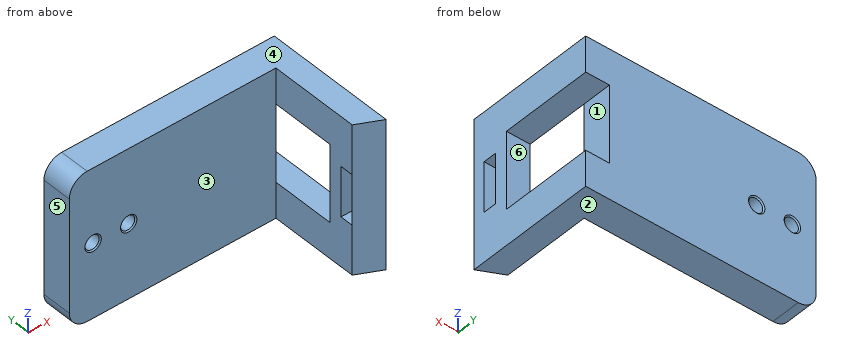
```python
from build123d import *

# Parameters (mm, degrees)
SKETCH1_W             = 44.196
SKETCH1_H             = 31.75
BOSS_EXTRUDE1_DEPTH   = 6.35
F_3_0MM_DOWEL_HOLE1_D = 3
CHAMFER1_SIZE         = 0.254
FILLET2_R             = 3.81
BOSS_EXTRUDE4_DEPTH   = 5.08
SKETCH7_W             = 10.668
SKETCH7_H             = 2.794
CUT_EXTRUDE1_DEPTH    = 58.656321561
SKETCH8_W             = 5.08
SKETCH8_H             = 31.75
BOSS_EXTRUDE5_DEPTH   = 2.54
CUT_EXTRUDE2_DEPTH    = 63.468510275
SKETCH10_W            = 5.08
SKETCH10_H            = 16.51
CUT_EXTRUDE3_DEPTH    = 2.032


with BuildPart() as part:
    # Sketch1 → Boss-Extrude1 (new body)
    with BuildSketch(Plane(origin=(0, 0, 0), x_dir=(1, 0, 0), z_dir=(0, 1, 0))):
        with Locations((22.098, 15.875)):
            Rectangle(SKETCH1_W, SKETCH1_H)
    extrude(amount=BOSS_EXTRUDE1_DEPTH)

    # Ø3.0mm Dowel Hole1 (through all)
    with Locations(Plane(origin=(0, 6.35, 0), x_dir=(1, 0, 0), z_dir=(0, 1, 0))):
        with Locations((5.08, 15.875), (12.7, 15.875)):
            Hole(F_3_0MM_DOWEL_HOLE1_D / 2)

    # Chamfer1
    chamfer1_edges = [part.edges().sort_by_distance(p)[0] for p in [
        (14.2, 6.35, -15.875),
        (14.2, 0, -15.875),
        (6.58, 6.35, -15.875),
        (6.58, 0, -15.875),
    ]]
    chamfer(chamfer1_edges, length=CHAMFER1_SIZE)

    # Fillet2
    fillet2_edges = [part.edges().sort_by_distance(p)[0] for p in [
        (0, 3.175, -31.75),
        (0, 3.175, 0),
    ]]
    fillet(fillet2_edges, radius=FILLET2_R)

    # Sketch6 → Boss-Extrude4 (add)
    with BuildSketch(Plane(origin=(44.196, 0, 0), x_dir=(0, 0, -1), z_dir=(1, 0, 0))):
        Polygon((0, 6.35), (0, -19.05), (31.75, -19.05), (31.75, 6.35), (24.13, 6.35), (24.13, -11.43), (7.62, -11.43), (7.62, 6.35), align=None)
    extrude(amount=BOSS_EXTRUDE4_DEPTH)

    # Sketch7 → Cut-Extrude1 (cut, through all)
    with BuildSketch(Plane.ZY.offset(-44.196)):
        with Locations((-15.875, -17.653)):
            Rectangle(SKETCH7_W, SKETCH7_H)
    extrude(amount=-CUT_EXTRUDE1_DEPTH, mode=Mode.SUBTRACT)

    # Sketch8 → Boss-Extrude5 (add)
    with BuildSketch(Plane.XZ.offset(19.05)):
        with Locations((46.736, -15.875)):
            Rectangle(SKETCH8_W, SKETCH8_H)
    extrude(amount=BOSS_EXTRUDE5_DEPTH)

    # Sketch9 → Cut-Extrude2 (cut, through all)
    with BuildSketch(Plane(origin=(0, 0, -31.75), x_dir=(-1, 0, 0), z_dir=(0, 0, -1))):
        Polygon((-49.276, -21.59), (-44.196, -19.05), (-44.196, -21.59), align=None)
    extrude(amount=-CUT_EXTRUDE2_DEPTH, mode=Mode.SUBTRACT)

    # Sketch10 → Cut-Extrude3 (cut)
    with BuildSketch(Plane(origin=(0, -11.43, 0), x_dir=(1, 0, 0), z_dir=(0, 1, 0))):
        with Locations((46.736, 15.875)):
            Rectangle(SKETCH10_W, SKETCH10_H)
    extrude(amount=-CUT_EXTRUDE3_DEPTH, mode=Mode.SUBTRACT)


solid = part.part
```
Source: CAD feature listing. Evaluate the final solid. Frame: model axes, mm. Face numbers are marked on the shaded views. A direction names the side the tool comes from. Give positions to 0.01 mm unless a question says otherwise; leave off trailing zeros. Order: outer loops, then holes, each group sorted by start corner. A loop starts at its lowest first (then second) coordinate and runs counter-clockwise, first axis right, second up.
(1) Pull-direction query (Z, two-part tool) for the marked faces 4, 5 and 6; classes: +Z half, -Z half, draft (parallel to the pull), parting line (faces both ways), or undercut.
(2) Section query A-A (x = 5.08). Return the cut outline in (y, z) (3 decimals).
(3) Material intervals for line 1 along Z through (x, y) = (5.08, 4.5) (3 decimals); line 2 along Z through (x, y) = (45, -17); line 3 along Y through (x, z) = (30, -26), sorted ascending.
(4) Section query D-D (x = 22). Return the cut outline in (y, z), plus the area to 3 significant figures.
(5) Access query for the marked faces 1, 2 and 3. Directions: +Z, -Z, +X, -X, +Y, -Y. A direction counts if a zero-diameter tool reaches every point of the face in a straight line with its end or side. Return the directions, or none.
(6) Section query B-B (y = -4.5). Return the cut outline in (x, z).
(7) Section query C-C (y = 2). Return the cut outline in (x, z) (3 decimals), plus the area to 3 significant figures.
(8) Contact query for flat-ended pins moving along their axis: P1, Ø7, axis at y = 2.5, z = -12, coming from the +X side; P2, Ø8, axis at x = 39, z = -28, coming from the -Y side; P3, Ø2.5, axis at x = 12.7, z = -15.875, coming from the -Y side; P4, Ø4, axis at y = -11.5, z = -10.5, coming from the -X side. Output: stop coordinate, or through.
Outcome:
1. face 4: +Z half
1. face 5: draft
1. face 6: undercut
2. outline: (0, -31.75) - (6.35, -31.75) - (6.35, -17.629) - (6.096, -17.375) - (0.254, -17.375) - (0, -17.629) - close; (0, -14.121) - (0.254, -14.375) - (6.096, -14.375) - (6.35, -14.121) - (6.35, 0) - (0, 0) - close
3. line 1: z = -31.75 to -17.375, -14.375 to 0
3. line 2: z = -31.75 to -21.21, -10.54 to 0
3. line 3: y = 0 to 6.35
4. outline: (0, -31.75) - (6.35, -31.75) - (6.35, 0) - (0, 0) - close
4. area: 202 mm2
5. face 1: +X, +Y
5. face 2: -Z, +X, -X, +Y, -Y
5. face 3: +Z, -Z, -X, -Y
6. outline: (44.2, -31.75) - (49.28, -31.75) - (49.28, -24.13) - (44.2, -24.13) - close; (44.2, -7.62) - (49.28, -7.62) - (49.28, 0) - (44.2, 0) - close
7. outline: (0, -27.94) arc R3.81 ccw to (3.81, -31.75) - (49.276, -31.75) - (49.276, -24.13) - (44.196, -24.13) - (44.196, -7.62) - (49.276, -7.62) - (49.276, 0) - (3.81, 0) arc R3.81 ccw to (0, -3.81) - close; hole circle Ø3 at (5.08, -15.875); hole circle Ø3 at (12.7, -15.875)
7. area: 1,460 mm2
8. P1: stops at x = 44.2
8. P2: stops at y = 0
8. P3: passes through
8. P4: stops at x = 44.2
